Could you check a few things on this model? Use its own coordinates, in mm. A direction names the side the tool comes from. Coordinates: 2 decimals unless noted, no trailing zeros. Order: outer loops, then holes, each group sorted by start corner. A loop starts at its lowest first (then second) coordinate and runs counter-clockwise, first axis right, second up. Notation, with made-up numbers: M 38.25,26 L 63.25,26 A17 ccw 63.25,58 Z; hole C -26,46 d8. An arc over 180 degrees is marked long. Write item = value, one per line. Start each with the question number.
from build123d import *

# Parameters (mm, degrees)
BOSS_EXTRUDE1_DEPTH = 35
SKETCH2_R           = 9
BOSS_EXTRUDE2_DEPTH = 2
SKETCH3_R           = 4
CUT_EXTRUDE1_DEPTH  = 5
SKETCH4_W           = 7.5
SKETCH4_H           = 35
BOSS_EXTRUDE3_DEPTH = 20.5
BOSS_EXTRUDE4_START = -7.5
SKETCH6_W           = 5
SKETCH6_H           = 25.5
BOSS_EXTRUDE4_DEPTH = 7.5
SKETCH7_W           = 5
SKETCH7_H           = 20
BOSS_EXTRUDE5_DEPTH = 7.5
SKETCH8_W           = 20
SKETCH8_H           = 5
BOSS_EXTRUDE6_DEPTH = 15
SKETCH10_W          = 16
SKETCH10_H          = 16
CUT_EXTRUDE2_DEPTH  = 7.5


with BuildPart() as part:
    # Sketch1 → Boss-Extrude1 (new body)
    with BuildSketch(Plane.XY):
        Polygon((-9.305574102, 4.73561153), (18.194425898, 4.73561153), (18.194425898, -0.26438847), (1.694425898, -0.26438847), (-4.305574102, -6.26438847), (-4.305574102, -13.26438847), (-9.305574102, -13.26438847), align=None)
    extrude(amount=BOSS_EXTRUDE1_DEPTH)

    # Sketch2 → Boss-Extrude2 (add)
    with BuildSketch(Plane(origin=(0, 4.73561153, 0), x_dir=(1, 0, 0), z_dir=(0, 1, 0))):
        with Locations((2.904425898, -17.63)):
            Circle(SKETCH2_R)
    extrude(amount=BOSS_EXTRUDE2_DEPTH)

    # Sketch3 → Cut-Extrude1 (cut)
    with BuildSketch(Plane(origin=(0, 6.73561153, 0), x_dir=(1, 0, 0), z_dir=(0, 1, 0))):
        with Locations((2.904425898, -17.63)):
            Circle(SKETCH3_R)
    extrude(amount=-CUT_EXTRUDE1_DEPTH, mode=Mode.SUBTRACT)

    # Sketch4 → Boss-Extrude3 (add)
    with BuildSketch(Plane.XZ.offset(0.26438847)):
        with Locations((14.444425898, 17.5)):
            Rectangle(SKETCH4_W, SKETCH4_H)
    extrude(amount=BOSS_EXTRUDE3_DEPTH)

    # Sketch6 → Boss-Extrude4 (add)
    with BuildSketch(Plane(origin=(18.194425898, 0, 0), x_dir=(0, 0, -1), z_dir=(1, 0, 0)).offset(BOSS_EXTRUDE4_START)):
        with Locations((-2.5, -8.01438847)):
            Rectangle(SKETCH6_W, SKETCH6_H)
    extrude(amount=BOSS_EXTRUDE4_DEPTH)

    # Sketch7 → Boss-Extrude5 (add)
    with BuildSketch(Plane.XZ.offset(13.26438847)):
        with Locations((-6.805574102, 25)):
            Rectangle(SKETCH7_W, SKETCH7_H)
    extrude(amount=BOSS_EXTRUDE5_DEPTH)

    # Sketch8 → Boss-Extrude6 (add)
    with BuildSketch(Plane(origin=(-4.305574102, 0, 0), x_dir=(0, 0, -1), z_dir=(1, 0, 0))):
        with Locations((-25, -18.26438847)):
            Rectangle(SKETCH8_W, SKETCH8_H)
    extrude(amount=BOSS_EXTRUDE6_DEPTH)

    # Sketch10 → Cut-Extrude2 (cut)
    with BuildSketch(Plane(origin=(18.194425898, 0, 0), x_dir=(0, 0, -1), z_dir=(1, 0, 0))):
        with Locations((-21, -5.26438847)):
            Rectangle(SKETCH10_W, SKETCH10_H)
    extrude(amount=-CUT_EXTRUDE2_DEPTH, mode=Mode.SUBTRACT)


solid = part.part
(1) Thinking about a two-plate mould opening in X: for faces 1 (the flat face through (10.694, 1, 21)), 2 (the flat face through (-4.306, -11, 17)), 3 (the flat face through (-7, -13.264, 7)), which applies, released by +X, released by -X, zero draft, split by the parting line, or undercut?
(2) Please list where these lines run through material, in increasing order: probe 1 along Z at (x, y) = (14.75, 0.25); probe 2 along X at (y, z) = (4.6, 17.63); probe 3 along Y at (x, z) = (16.25, 25). Write a range as from..to.
(3) Imagine slicing it at A-A on y = -15. List the corners of the cut face in (x, z) for me, plus the area to 4 significant figures.
(4) Will these pins go through, and if not, where does the flat tip stop? P1, Ø7, axis at x = 2.9, z = 17.63, coming from the +Y side; P2, Ø4.5, axis at x = 4, z = 11, coming from the -Y side; P3, Ø1.5, axis at x = -6.5, z = 9, coming from the -Y side.
(5) Imagine slicing it at B-B on x = 5. List the corners of the cut face in (y, z) for me.
(6) Imagine slicing it at C-C on z = 17.63. List the corners of the cut face in (x, y) for me, plus the area to 3 significant figures.
(7) Imagine slicing it at D-D on y = -2. List the corners of the cut face in (x, z) for me, plus the area to 3 significant figures.
(8) For faces 4 (the flat face through (3, -15.764, 25)), 5 (the flat face through (14, -13.264, 21)), 6 (the flat face through (1, -18, 15)), 7 (the flat face through (-9.306, -5, 17)), 8 (the flat face through (3, 1.736, 18)), which set-ups out of +Z, -Z, +X, -X, +Y, -Y let a thin tool reach every point of the face, with its end or its side?
Response:
q1.face_1 = released by +X
q1.face_2 = undercut
q1.face_3 = zero draft
q2.probe_1 = 0..13, 29..35
q2.probe_2 = -9.31..-1.1, 6.9..18.19
q2.probe_3 = -20.76..-13.26, 2.74..4.74
q3.outline = M -9.31,15 L -4.31,15 L -4.31,35 L -9.31,35 Z; M 10.69,0 L 18.19,0 L 18.19,35 L 10.69,35 Z
q3.area = 362.5 mm2
q4.P1 = 1.74
q4.P2 = -0.26
q4.P3 = -13.26
q5.outline = M -20.76,15 L -15.76,15 L -15.76,35 L -20.76,35 Z; M -0.26,0 L 4.74,0 L 4.74,8.88 L 6.74,8.88 L 6.74,14.22 L 1.74,14.22 L 1.74,21.04 L 6.74,21.04 L 6.74,26.38 L 4.74,26.38 L 4.74,35 L -0.26,35 Z
q6.outline = M -9.31,-20.76 L 18.19,-20.76 L 18.19,-13.26 L 10.69,-13.26 L 10.69,-15.76 L -4.31,-15.76 L -4.31,-6.26 L 1.69,-0.26 L 10.69,-0.26 L 10.69,2.74 L 18.19,2.74 L 18.19,4.74 L 11.9,4.74 L 11.9,6.74 L 6.9,6.74 L 6.9,1.74 L -1.1,1.74 L -1.1,6.74 L -6.1,6.74 L -6.1,4.74 L -9.31,4.74 Z
q6.area = 363 mm2
q7.outline = M -9.31,0 L -0.04,0 L -0.04,35 L -9.31,35 Z; M 10.69,0 L 18.19,0 L 18.19,13 L 10.69,13 Z; M 10.69,29 L 18.19,29 L 18.19,35 L 10.69,35 Z
q7.area = 467 mm2
q8.face_4 = +Z, -Z
q8.face_5 = +X
q8.face_6 = -Z, -X, -Y
q8.face_7 = +Z, -Z, -X, +Y, -Y
q8.face_8 = +Y
